Autodesk Inventor part; units mm, degrees
ref_plane "YZ Plane" through (0, 0, 0) normal (1, 0, 0) x (0, 1, 0)
ref_plane "XZ Plane" through (0, 0, 0) normal (0, 1, 0) x (-1, 0, 0)
ref_plane "XY Plane" through (0, 0, 0) normal (0, 0, 1) x (1, 0, 0)
sketch "Sketch1" plane through (0, 0, 0) normal (1, 0, 0) x (0, 1, 0)
  line L0 (74.1326, 23.8494) -> (-27.4674, 23.8494)
  line L1 (-27.4674, 23.8494) -> (-27.4674, -26.9506)
  line L2 (-27.4674, -26.9506) -> (74.1326, -26.9506)
  line L3 (74.1326, -26.9506) -> (74.1326, 23.8494)
  point P0 (0, 0)
  dimension "d0" = 50.8
  dimension "d1" = 101.6
extrude "Extrusion1" add sketch "Sketch1" along normal blind 9.525
sketch "Sketch2" plane through (9.525, 0, 0) normal (1, 0, 0) x (0, 0, -1)
  line L0 (-23.8494, 74.1326) -> (-23.8494, -27.4674)
  line L1 (26.9506, 74.1326) -> (-23.8494, 74.1326)
  point P0 (0, 0)
  point P1 (1.5506, 61.4326)
  dimension "d11" = 25.4
  dimension "d12" = 12.7
hole "Hole1" at (9.525, 61.4326, -1.5506) direction (-1, 0, 0) diameter 6.7564 end through all counterbore diameter 12.7 counterbore depth 3.175
sketch "Sketch3" plane through (9.525, 0, 0) normal (1, 0, 0) x (0, 0, -1)
  line L0 (-23.8494, 74.1326) -> (-23.8494, -27.4674)
  line L1 (-23.8494, -27.4674) -> (26.9506, -27.4674)
  point P0 (0, 0)
  point P1 (1.5506, -14.7674)
  dimension "d21" = 25.4
  dimension "d22" = 12.7
hole "Hole2" at (9.525, -14.7674, -1.5506) direction (-1, 0, 0) diameter 6.7564 end through all counterbore diameter 12.7 counterbore depth 3.175
sketch "Sketch4" plane through (0, 0, 0) normal (-1, 0, 0) x (0, 0, 1)
  line L0 (-26.9506, 74.1326) -> (23.8494, 74.1326)
  line L1 (23.8494, 74.1326) -> (23.8494, -27.4674)
  point P0 (0, 0)
  point P1 (8.7364, 40.8586)
  dimension "d30" = 33.274
  dimension "d31" = 15.113
hole "Hole3" at (0, 40.8586, 8.7364) direction (1, 0, 0) diameter 2.159 end through all counterbore diameter 5.08 counterbore depth 1.651
sketch "Sketch5" plane through (0, 0, 0) normal (-1, 0, 0) x (0, 0, 1)
  line L0 (23.8494, -27.4674) -> (-26.9506, -27.4674)
  line L1 (-26.9506, 74.1326) -> (23.8494, 74.1326)
  line L2 (23.8494, 74.1326) -> (23.8494, -27.4674)
  point P0 (0, 0)
  point P1 (8.7364, 5.8066)
  dimension "d41" = 33.274
  dimension "d42" = 15.113
hole "Hole4" at (0, 5.8066, 8.7364) direction (1, 0, 0) diameter 2.159 end through all counterbore diameter 5.08 counterbore depth 1.651
sketch "Sketch6" plane through (0, 0, 0) normal (-1, 0, 0) x (0, 0, 1)
  line L0 (-26.9506, -27.4674) -> (-26.9506, 74.1326)
  line L1 (-26.9506, 74.1326) -> (23.8494, 74.1326)
  point P0 (0, 0)
  point P1 (-11.8376, 40.8586)
  dimension "d50" = 15.113
  dimension "d51" = 33.274
hole "Hole5" at (0, 40.8586, -11.8376) direction (1, 0, 0) diameter 2.159 end through all counterbore diameter 5.08 counterbore depth 1.651
sketch "Sketch7" plane through (0, 0, 0) normal (-1, 0, 0) x (0, 0, 1)
  line L0 (-26.9506, -27.4674) -> (-26.9506, 74.1326)
  line L1 (23.8494, -27.4674) -> (-26.9506, -27.4674)
  point P0 (0, 0)
  point P1 (-11.8376, 5.8066)
  dimension "d59" = 15.113
  dimension "d60" = 33.274
hole "Hole6" at (0, 5.8066, -11.8376) direction (1, 0, 0) diameter 2.159 end through all counterbore diameter 5.08 counterbore depth 1.651
properties part number "FV mounting plate V1"
Design review of the part built by this model. Coordinates are the model's own, in mm. A direction names the side the tool comes from. Give positions to 0.01 mm unless a question says otherwise; leave off trailing zeros. Order: outer loops, then holes, each group sorted by start corner. A loop starts at its lowest first (then second) coordinate and runs counter-clockwise, first axis right, second up.
1. Add section B-B, the plane y = 56. State the section outline as (x, z) points (3 decimals), then the cut area to 3 significant figures.
Solution:
outline: (0, -26.951) - (9.525, -26.951) - (9.525, -4.838) - (6.35, -4.838) - (6.35, 1.737) - (9.525, 1.737) - (9.525, 23.849) - (0, 23.849) - close
area: 463 mm2
2. Mouldability with a two-part tool opening along Z and no side actions: class faces 4 (the flat face through (5, 24, 23.849)), 5 (the flat face through (5, 74.133, -2)), 6 (the cylindrical face through (0.84, 38.34, 8.41)) as +Z half, -Z half, draft (parallel to the pull), parting line (faces both ways), or undercut.
Solution:
face 4: +Z half
face 5: draft
face 6: undercut
3. Add section C-C, the plane x = 3.75. State the section outline as (y, z) points.
Solution:
outline: (-27.47, -26.95) - (74.13, -26.95) - (74.13, 23.85) - (-27.47, 23.85) - close; hole circle Ø6.76 at (-14.77, -1.55); hole circle Ø2.16 at (5.81, -11.84); hole circle Ø2.16 at (5.81, 8.74); hole circle Ø2.16 at (40.86, -11.84); hole circle Ø2.16 at (40.86, 8.74); hole circle Ø6.76 at (61.43, -1.55)
4. Add section A-A, the plane z = -1. State the section outline as (x, y) points (3 decimals), then the cut area to 3 significant figures.
Solution:
outline: (0, -27.467) - (9.525, -27.467) - (9.525, -21.093) - (6.35, -21.093) - (6.35, -18.1) - (0, -18.1) - close; (0, -11.434) - (6.35, -11.434) - (6.35, -8.441) - (9.525, -8.441) - (9.525, 55.107) - (6.35, 55.107) - (6.35, 58.1) - (0, 58.1) - close; (0, 64.766) - (6.35, 64.766) - (6.35, 67.759) - (9.525, 67.759) - (9.525, 74.133) - (0, 74.133) - close
area: 803 mm2
5. For pin 1 Ø2.5 at (y, z) = (40.5, -11.5) entering from -X; pin 2 Ø6.5 at (y, z) = (62, -3.5) entering from +X; pin 3 Ø1.9 at (y, z) = (5.81, -11.84) entering from -X, all flat-tipped, find the tip position at first contact; note any pin that passes through.
Solution:
pin 1: stops at x = 1.65
pin 2: stops at x = 6.35
pin 3: passes through
6. Add section D-D, the plane y = -16. State the section outline as (x, z) points (3 decimals).
Solution:
outline: (0, -26.951) - (9.525, -26.951) - (9.525, -7.78) - (6.35, -7.78) - (6.35, -4.696) - (0, -4.696) - close; (0, 1.595) - (6.35, 1.595) - (6.35, 4.679) - (9.525, 4.679) - (9.525, 23.849) - (0, 23.849) - close
7. Tool access review of faces 1 (the flat face through (6.35, -12, -4)), 2 (the flat face through (1.651, 6, 10)), 3 (the flat face through (9.525, 23, -1)): name each direction out of +Z, -Z, +X, -X, +Y, -Y from which nothing blocks a thin tool from reaching the whole face with its end or side.
Solution:
face 1: +X
face 2: -X
face 3: +Z, -Z, +X, +Y, -Y
8. To check wall thickness, follow L1, parallel to Y at x = 6.25, z = -0.5; L2, parallel to Z at x = 0.5, y = 60.5; L3, parallel to Y at x = 1.75, z = 9. State the ranges of each line that lie inside material, in increasing order.
Solution:
L1: y = -27.47 to -17.98, -11.56 to 58.22, 64.64 to 74.13
L2: z = -26.95 to -4.8, 1.7 to 23.85
L3: y = -27.47 to 4.76, 6.85 to 39.81, 41.91 to 74.13
